Design review of the part shown in the three views and the two pictorial views. Dimensions are in mm from the part's minimum x, y and z. A direction names the side the tool comes from. Round coordinates to 2 decimals unless told otherwise and drop trailing zeros. Write each loop counter-clockwise with the first axis right and the second up, starting at its lowest first coordinate (ties: lowest second). Pieces come first, ordered by that corner, then holes. Notation, with made-up numbers: (89, 8) -> (110, 8) arc R16 cw to (110, 36) -> close; hole circle Ø11 at (63, 34.25). An arc over 180 degrees is marked (long way). One line per question, with ' | ' between items. Start each with the question number.
1) Insertion check: pin 1 Ø10 at (x, y) = (35.5, 100) entering from +Z; pin 2 Ø8 at (x, z) = (134.5, 62) entering from -Y; pin 3 Ø12 at (x, y) = (55.5, 37) entering from +Z. Each pin has a flat end and moves straight along its axis. Give the tip position at first contact, or say it passes through.
2) For the marked faces 1 and 2, list the 3-axis set-ups (+Z, -Z, +X, -X, +Y, -Y) from which the entire face can be reached by the end or side of a thin tool; tool diameter is ignored.
3) Consider section B-B (z = 30.5). Give the boundary of the cut face in (x, y) (1 decimal).
4) Consider section C-C (z = 40.5). Give the boundary of the cut face in (x, y) (1 decimal).
5) Consider section A-A (x = 106). Give the boundary of the cut face in (y, z), then the cut area to 3 significant figures.
6) Consider section D-D (x = 47). Give the boundary of the cut face in (y, z) (1 decimal), then the cut area to 3 significant figures.
7) For probe 1 along Y at (x, z) = (152, 43); probe 2 along X at (y, z) = (16, 42); probe 3 along X at (y, z) = (134, 54.5) (1 decimal), list the stretches that pass through material, from the lowest coordinate up.
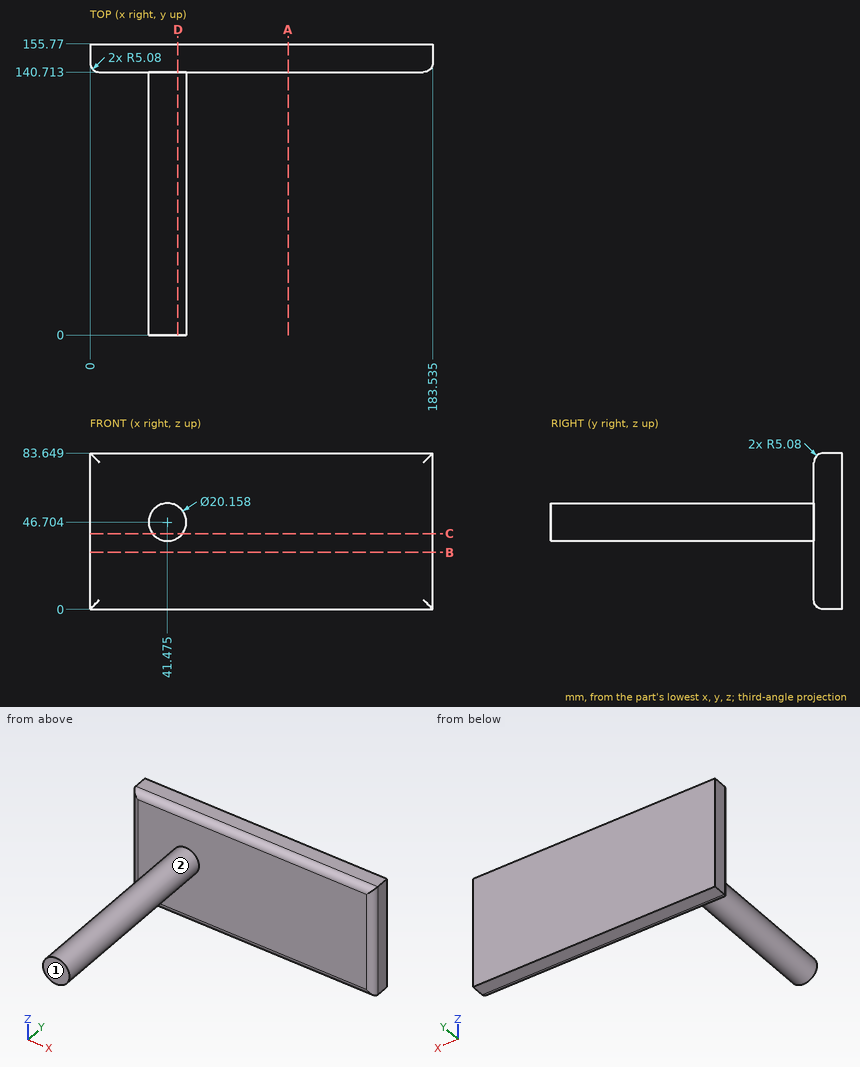
From the geometry:
1) pin 1: stops at z = 56.74 | pin 2: stops at y = 140.71 | pin 3: stops at z = 52.8
2) face 1: +Z, -Z, +X, -X, -Y | face 2: -Y
3) outline: (0, 145.8) arc R5.1 ccw to (5.1, 140.7) -> (178.5, 140.7) arc R5.1 ccw to (183.5, 145.8) -> (183.5, 155.8) -> (0, 155.8) -> close
4) outline: (0, 145.8) arc R5.1 ccw to (5.1, 140.7) -> (33.5, 140.7) -> (33.5, 0) -> (49.4, 0) -> (49.4, 140.7) -> (178.5, 140.7) arc R5.1 ccw to (183.5, 145.8) -> (183.5, 155.8) -> (0, 155.8) -> close
5) outline: (140.71, 5.08) arc R5.08 ccw to (145.79, 0) -> (155.77, 0) -> (155.77, 83.65) -> (145.79, 83.65) arc R5.08 ccw to (140.71, 78.57) -> close | area: 1,250 mm2
6) outline: (0, 38.3) -> (140.7, 38.3) -> (140.7, 5.1) arc R5.1 ccw to (145.8, 0) -> (155.8, 0) -> (155.8, 83.6) -> (145.8, 83.6) arc R5.1 ccw to (140.7, 78.6) -> (140.7, 55.1) -> (0, 55.1) -> close | area: 3,620 mm2
7) probe 1: y = 140.71 to 155.77 | probe 2: x = 32.56 to 50.39 | probe 3: x = 35.1 to 47.9
